CAD build for the part. Positions are in the model's coordinates, mm. Give positions to 0.01 mm unless a question says otherwise; leave off trailing zeros. Write each loop counter-clockwise with the first axis right and the second up, starting at its lowest first coordinate (ties: lowest second). Pieces come first, ordered by that corner, then holes. Notation, with made-up numbers: (-4.75, 48.5) -> (38.25, 48.5) arc R18 cw to (38.25, 63.5) -> close; hole circle Ø8 at (-13, 32). An arc over 180 degrees is marked (long way). Use one line per item in the form item = value. Start each with the question number.
from build123d import *

# Parameters (mm, degrees)
SKETCH1_W           = 6
SKETCH1_H           = 50
SKETCH1_W_2         = 50
SKETCH1_H_2         = 6
BOSS_EXTRUDE1_DEPTH = 6


with BuildPart() as part:
    # Sketch1 → Boss-Extrude1 (new body)
    with BuildSketch(Plane(origin=(0, 0, 0), x_dir=(0, 0, -1), z_dir=(1, 0, 0))):
        with BuildLine():
            Line((-414.831767264, 357.151199882), (3.168232736, 357.151199882))
            ThreePointArc((3.168232736, 357.151199882), (73.878910855, 327.861878001), (103.168232736, 257.151199882))
            Line((103.168232736, 257.151199882), (103.168232736, -324.848800118))
            Line((103.168232736, -324.848800118), (-414.831767264, -324.848800118))
            Line((-414.831767264, -324.848800118), (-414.831767264, 357.151199882))
        make_face()
        with Locations((-405.831767264, 272.151199882)):
            Rectangle(SKETCH1_W, SKETCH1_H, mode=Mode.SUBTRACT)
        with Locations((-253.831767264, -315.848800118)):
            Rectangle(SKETCH1_W_2, SKETCH1_H_2, mode=Mode.SUBTRACT)
        with Locations((-57.831767264, -315.848800118)):
            Rectangle(SKETCH1_W_2, SKETCH1_H_2, mode=Mode.SUBTRACT)
        with Locations((-253.831767264, -159.848800118)):
            Rectangle(SKETCH1_W_2, SKETCH1_H_2, mode=Mode.SUBTRACT)
        with Locations((-57.831767264, -159.848800118)):
            Rectangle(SKETCH1_W_2, SKETCH1_H_2, mode=Mode.SUBTRACT)
        with Locations((-253.831767264, -3.848800118)):
            Rectangle(SKETCH1_W_2, SKETCH1_H_2, mode=Mode.SUBTRACT)
        with Locations((-57.831767264, -3.848800118)):
            Rectangle(SKETCH1_W_2, SKETCH1_H_2, mode=Mode.SUBTRACT)
        with Locations((-253.831767264, 152.151199882)):
            Rectangle(SKETCH1_W_2, SKETCH1_H_2, mode=Mode.SUBTRACT)
        with Locations((-57.831767264, 152.151199882)):
            Rectangle(SKETCH1_W_2, SKETCH1_H_2, mode=Mode.SUBTRACT)
        with Locations((-405.831767264, -239.848800118)):
            Rectangle(SKETCH1_W, SKETCH1_H, mode=Mode.SUBTRACT)
    extrude(amount=BOSS_EXTRUDE1_DEPTH)


solid = part.part
1) Wall check: line 1 along Y through (x, z) = (0.35, 80); line 2 along Z through (x, y) = (1.3, -243.5); line 3 along Y through (x, z) = (5.15, -31.5). Give the ranges that are in metal, low to high. Write a range as from..to.
2) Cut at A-A (z = 68.5). Give the cut face in (x, y), and give its area (3 significant figures).
3) Cut at B-B (y = 277). Give the cut face in (x, z).
4) Pin check, flat tips, straight feed: pin 1 (1.5 mm diameter, centred on y = 227.5, z = 12.5, fed in from -X); pin 2 (3 mm diameter, centred on x = 1.5, y = 265, fed in from -Z). Stop position of each tip, or through.
Final values:
q1.line_1 = -324.85..-318.85, -312.85..-162.85, -156.85..-6.85, -0.85..149.15, 155.15..357.15
q1.line_2 = -103.17..402.83, 408.83..414.83
q1.line_3 = -324.85..353.05
q2.outline = (0, -324.85) -> (6, -324.85) -> (6, -318.85) -> (0, -318.85) -> close; (0, -312.85) -> (6, -312.85) -> (6, -162.85) -> (0, -162.85) -> close; (0, -156.85) -> (6, -156.85) -> (6, -6.85) -> (0, -6.85) -> close; (0, -0.85) -> (6, -0.85) -> (6, 149.15) -> (0, 149.15) -> close; (0, 155.15) -> (6, 155.15) -> (6, 357.15) -> (0, 357.15) -> close
q2.area = 3,950 mm^2
q3.outline = (0, -101.18) -> (6, -101.18) -> (6, 402.83) -> (0, 402.83) -> close; (0, 408.83) -> (6, 408.83) -> (6, 414.83) -> (0, 414.83) -> close
q4.pin_1 = 0
q4.pin_2 = -102.97
